Design review of the part built by this model. Coordinates are the model's own, in mm. A direction names the side the tool comes from. Round coordinates to 2 decimals unless told otherwise and drop trailing zeros. Loops run counter-clockwise (first coordinate to the right, second up) from the corner with the lowest first, then second, coordinate; pieces in that order, holes last. Notation, with made-up numbers: (4, -8.75) - (57, -8.75) arc R10 cw to (57, 8.25) - close; hole circle Ø4 at (60, -35.5). An arc over 180 degrees is marked (long way). Answer as CSV lines item,"result". Start each with the question number.
(1) Mouldability with a two-part tool opening along X and no side actions: class faces 1 (the flat face through (-21, -40, 25)), 2 (the cylindrical face through (-11.923, -53.692, 23.732)), 3 (the flat face through (9, -9, 24)) as released by +X, released by -X, zero draft, split by the parting line, or undercut.
(2) Consider section A-A (z = 6.75). Give the boundary of the cut face in (x, y), and give its area (3 significant figures).
(3) For P1, Ø8, axis at x = -16, z = 8.5, coming from the +Y side; P2, Ø5, axis at y = 23, z = 15.5, coming from the -X side; P3, Ø3, axis at y = 18, z = 11, coming from the -X side, all flat-tipped, find the tip position at first contact; note any pin that passes through.
(4) Wall thickness on L1, parallel to Z at x = -11, y = -50; L2, parallel to Y at x = 0, z = 9.5; L3, parallel to Z at x = 0, y = -36: over which ranges is each line inside the solid? List them lowest first.
(5) For faces 4 (the cylindrical face through (47.69, -15.02, 12.36)), 5 (the cylindrical face through (-11.923, -53.692, 1.232)), 6 (the flat face through (9, -9, 1)), list the 3-axis set-ups (+Z, -Z, +X, -X, +Y, -Y) from which the entire face can be reached by the end or side of a thin tool; tool diameter is ignored.
from build123d import *

# Parameters (mm, degrees)
CROQUIS1_R                 = 55
CROQUIS1_R_2               = 6
SALIENTE_EXTRUIR1_DEPTH    = 25
CROQUIS3_W                 = 20
CROQUIS3_H                 = 10
CROQUIS4_R                 = 45
CROQUIS4_R_2               = 10
CORTAR_EXTRUIR1_DEPTH      = 1
CHAFL_N1_SIZE              = 1
CHAFL_N1_OF_SIMETR_A2_SIZE = 1


with BuildPart() as part:
    # Croquis1 → Saliente-Extruir1 (new body)
    with BuildSketch(Plane.XY):
        Circle(CROQUIS1_R)
        Circle(CROQUIS1_R_2, mode=Mode.SUBTRACT)
    extrude(amount=SALIENTE_EXTRUIR1_DEPTH)

    # Croquis3 → Cortar-Revolución1 (revolve, cut)
    with BuildSketch(Plane(origin=(0, 0, 0), x_dir=(0, 0, -1), z_dir=(1, 0, 0)), mode=Mode.PRIVATE) as cortar_revoluci_n1_sk:
        with Locations((-12.5, 55)):
            Rectangle(CROQUIS3_W, CROQUIS3_H)
    revolve(cortar_revoluci_n1_sk.sketch.rotate(Axis((0, 0, 25), (0, 0, -1)), 90), axis=Axis((0, 0, 25), (0, 0, -1)), mode=Mode.SUBTRACT)

    # Croquis4 → Cortar-Extruir1 (cut)
    with BuildSketch(Plane.XY.offset(25)):
        Circle(CROQUIS4_R)
        Circle(CROQUIS4_R_2, mode=Mode.SUBTRACT)
    cortar_extruir1 = extrude(amount=-CORTAR_EXTRUIR1_DEPTH, mode=Mode.SUBTRACT)

    # Chaflán1
    chafl_n1_edges = [part.edges().sort_by_distance(p)[0] for p in [
        (-45, 0, 24),
        (-10, 0, 24),
    ]]
    chamfer(chafl_n1_edges, length=CHAFL_N1_SIZE - 0.0001)  # a hair under: the kernel refuses the full size

    # Simetría2: Cortar-Extruir1 across plane
    add(cortar_extruir1.mirror(Plane.XY.offset(12.5)), mode=Mode.SUBTRACT)

    # Chaflán1 of Simetría2
    chafl_n1_of_simetr_a2_edges = [part.edges().sort_by_distance(p)[0] for p in [
        (-45, 0, 1),
        (-10, 0, 1),
    ]]
    chamfer(chafl_n1_of_simetr_a2_edges, length=CHAFL_N1_OF_SIMETR_A2_SIZE - 0.0001)  # a hair under: the kernel refuses the full size


solid = part.part
Determined:
1,face 1,"zero draft"
1,face 2,"split by the parting line"
1,face 3,"undercut"
2,outline,"circle Ø100 at (0, 0); hole circle Ø12 at (0, 0)"
2,area,"7,740 mm^2"
3,P1,"stops at y = 48.54"
3,P2,"stops at x = -45.6"
3,P3,"stops at x = -47.2"
4,L1,"z = 0 to 2.5, 22.5 to 25"
4,L2,"y = -50 to -6, 6 to 50"
4,L3,"z = 1 to 24"
5,face 4,"none"
5,face 5,"+Z, -Z"
5,face 6,"-Z"
